For this review, use the dimensioned drawing (mm, ordinates from the lowest corner) and the shaded views. A direction names the side the tool comes from. Give positions to 0.01 mm unless a question says otherwise; leave off trailing zeros. Write each loop counter-clockwise with the first axis right and the second up, starting at its lowest first coordinate (ties: lowest second). Pieces come first, ordered by that corner, then holes.
1) We need section D-D on x = 40.4. Give the boundary of the cut face in (y, z), and give its area (3 significant figures).
2) Machinability: for the marked faces 1 and 2, which of the approach directions +Z, -Z, +X, -X, +Y, -Y give a long, thin tool a straight path to every point of the face, cutting with its end or side? Answer none if there is none.
3) We need section B-B on y = 6.75. Give the boundary of the cut face in (x, z).
4) Wall thickness on line 1 along Y through (x, z) = (40.4, 12); line 2 along X through (y, z) = (5.5, 12.75); line 3 along Z through (x, y) = (27, 20): over which ranges is each line inside the solid? List them lowest first.
5) We need section A-A on x = 17.5. Give the boundary of the cut face in (y, z).
6) We need section C-C on z = 3.75. Give the boundary of the cut face in (x, y).
7) Draft analysis for pull direction X (two halves, no side actions). For the marked faces 3, 4, 5 and 6, state which applies: pulls with the +X half, pulls with the -X half, needs draft (parallel to the pull), parting line crosses it, or undercut.
8) For P1, Ø6.5, axis at x = 5, y = 19.7, coming from the -Z side, flat-tipped, find the tip position at first contact; note if it passes through.
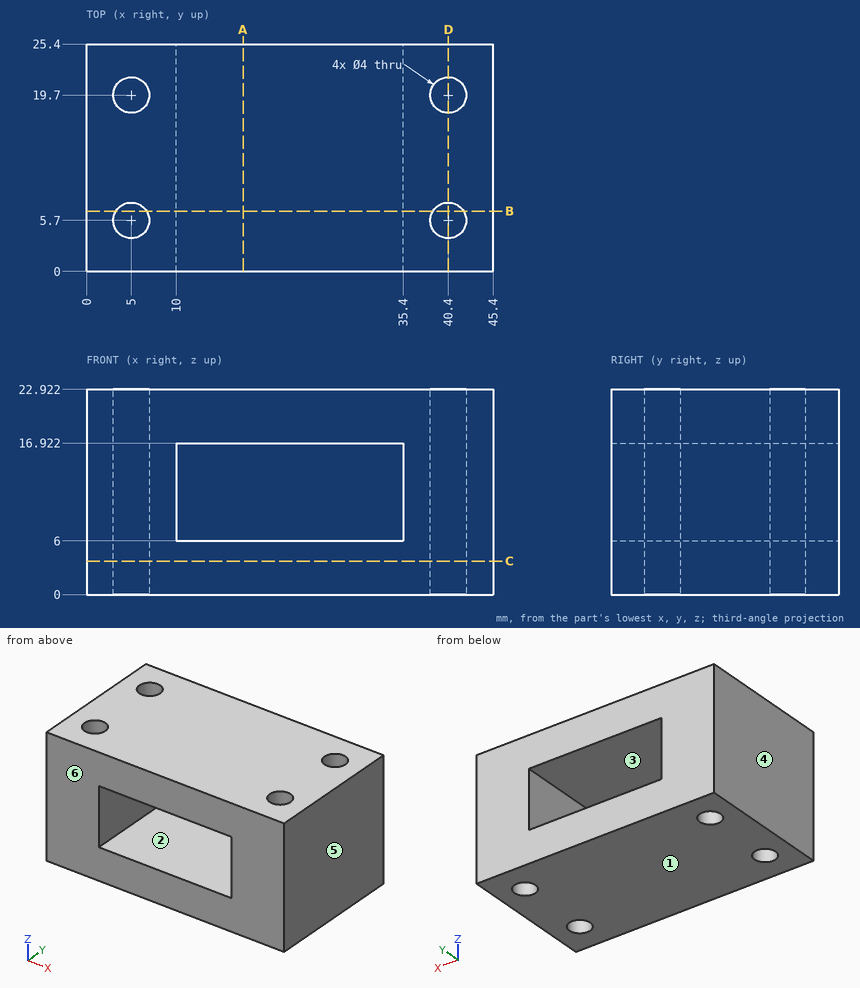
Results list:
1. outline: (0, 0) - (3.7, 0) - (3.7, 22.92) - (0, 22.92) - close; (7.7, 0) - (17.7, 0) - (17.7, 22.92) - (7.7, 22.92) - close; (21.7, 0) - (25.4, 0) - (25.4, 22.92) - (21.7, 22.92) - close
1. area: 399 mm2
2. face 1: -Z, +X, -X, +Y, -Y
2. face 2: +Y, -Y
3. outline: (0, 0) - (3.3, 0) - (3.3, 22.92) - (0, 22.92) - close; (6.7, 0) - (38.7, 0) - (38.7, 22.92) - (6.7, 22.92) - close; (42.1, 0) - (45.4, 0) - (45.4, 22.92) - (42.1, 22.92) - close; hole (10, 6) - (35.4, 6) - (35.4, 16.92) - (10, 16.92) - close
4. line 1: y = 0 to 3.7, 7.7 to 17.7, 21.7 to 25.4
4. line 2: x = 0 to 3.01, 6.99 to 10, 35.4 to 38.41, 42.39 to 45.4
4. line 3: z = 0 to 6, 16.92 to 22.92
5. outline: (0, 0) - (25.4, 0) - (25.4, 6) - (0, 6) - close; (0, 16.92) - (25.4, 16.92) - (25.4, 22.92) - (0, 22.92) - close
6. outline: (0, 0) - (45.4, 0) - (45.4, 25.4) - (0, 25.4) - close; hole circle Ø4 at (5, 5.7); hole circle Ø4 at (5, 19.7); hole circle Ø4 at (40.4, 5.7); hole circle Ø4 at (40.4, 19.7)
7. face 3: undercut
7. face 4: pulls with the -X half
7. face 5: pulls with the +X half
7. face 6: needs draft
8. P1: stops at z = 0
